Verification items for the finished model (mm, model axes). A direction names the side the tool comes from. Give positions to 0.01 mm unless a question says otherwise; leave off trailing zeros. Order: outer loops, then holes, each group sorted by start corner. A loop starts at its lowest first (then second) coordinate and runs counter-clockwise, first axis right, second up. Notation, with made-up numbers: M 61,79.5 L 98,79.5 A5 cw 98,87.5 Z; hole C -14,-33 d4. An arc over 180 degrees is marked long. Answer as a JSON object with one key per item and string values.
```python
from build123d import *

# Parameters (mm, degrees)
CROQUIS_TAPA_W                    = 110
CROQUIS_TAPA_H                    = 65
TAPA_DEPTH                        = 2.5
CROQUIS_PESTANA_W                 = 104.4
CROQUIS_PESTANA_H                 = 59.4
PESTANA_DEPTH                     = 4
CROQUIS_PESTANA_HUECO_W           = 101.4
CROQUIS_PESTANA_HUECO_H           = 56.4
PESTANA_HUECO_DEPTH               = 4
CROQUIS_POSTES_R                  = 2.5
POSTES_PCB_DEPTH                  = 29.9
VENTANA_LDR_Y_VENTILAS_DEPTH      = 71.535522965
VENTANA_LDR_Y_VENTILAS_DEPTH_BACK = 71.535522965
CROQUIS_VENTANA_Y_VENTILAS_R      = 3.5


with BuildPart() as part:
    # Croquis_tapa → Tapa (new body)
    with BuildSketch(Plane(origin=(0, 0, 0), x_dir=(1, 0, 0), z_dir=(0, 1, 0))):
        Rectangle(CROQUIS_TAPA_W, CROQUIS_TAPA_H)
    extrude(amount=TAPA_DEPTH)

    # Croquis_pestana → Pestana (add)
    with BuildSketch(Plane(origin=(0, 0, 0), x_dir=(1, 0, 0), z_dir=(0, 1, 0))):
        Rectangle(CROQUIS_PESTANA_W, CROQUIS_PESTANA_H)
    extrude(amount=-PESTANA_DEPTH)

    # Croquis_pestana_hueco → Pestana_hueco (cut)
    with BuildSketch(Plane(origin=(0, 0, 0), x_dir=(1, 0, 0), z_dir=(0, 1, 0))):
        Rectangle(CROQUIS_PESTANA_HUECO_W, CROQUIS_PESTANA_HUECO_H)
    extrude(amount=-PESTANA_HUECO_DEPTH, mode=Mode.SUBTRACT)

    # Croquis_postes → Postes_PCB (add)
    with BuildSketch(Plane(origin=(0, 0, 0), x_dir=(1, 0, 0), z_dir=(0, 1, 0))):
        with Locations(Location((-41, 22, 0), (0, 0, 270))):
            Circle(CROQUIS_POSTES_R)
        with Locations(Location((-41, -22, 0), (0, 0, 270))):
            Circle(CROQUIS_POSTES_R)
        with Locations(Location((41, 22, 0), (0, 0, 270))):
            Circle(CROQUIS_POSTES_R)
        with Locations(Location((41, -22, 0), (0, 0, 270))):
            Circle(CROQUIS_POSTES_R)
    extrude(amount=-POSTES_PCB_DEPTH)

    # Croquis_ventana_y_ventilas → Ventana_LDR_y_ventilas (cut, two sides: drawn at the far end of the back side and taken through both)
    with BuildSketch(Plane(origin=(0, 0, 0), x_dir=(1, 0, 0), z_dir=(0, 1, 0)).offset(-VENTANA_LDR_Y_VENTILAS_DEPTH_BACK)):
        with Locations(Location((33.46, -11, 0), (0, 0, 90))):
            Circle(CROQUIS_VENTANA_Y_VENTILAS_R)
        with BuildLine():
            Line((30, 0), (30, 8.68))
            ThreePointArc((30, 8.68), (31, 9.68), (32, 8.68))
            Line((32, 8.68), (32, 0))
            ThreePointArc((32, 0), (31, -1), (30, 0))
        make_face()
        with BuildLine():
            Line((34, 0), (34, 8.68))
            ThreePointArc((34, 8.68), (35, 9.68), (36, 8.68))
            Line((36, 8.68), (36, 0))
            ThreePointArc((36, 0), (35, -1), (34, 0))
        make_face()
        with BuildLine():
            Line((38, 0), (38, 8.68))
            ThreePointArc((38, 8.68), (39, 9.68), (40, 8.68))
            Line((40, 8.68), (40, 0))
            ThreePointArc((40, 0), (39, -1), (38, 0))
        make_face()
        with BuildLine():
            Line((-19, -15), (-19, 15))
            ThreePointArc((-19, 15), (-18, 16), (-17, 15))
            Line((-17, 15), (-17, -15))
            ThreePointArc((-17, -15), (-18, -16), (-19, -15))
        make_face()
        with BuildLine():
            Line((-23, -15), (-23, 15))
            ThreePointArc((-23, 15), (-22, 16), (-21, 15))
            Line((-21, 15), (-21, -15))
            ThreePointArc((-21, -15), (-22, -16), (-23, -15))
        make_face()
        with BuildLine():
            Line((-27, -15), (-27, 15))
            ThreePointArc((-27, 15), (-26, 16), (-25, 15))
            Line((-25, 15), (-25, -15))
            ThreePointArc((-25, -15), (-26, -16), (-27, -15))
        make_face()
        with BuildLine():
            Line((-31, -15), (-31, 15))
            ThreePointArc((-31, 15), (-30, 16), (-29, 15))
            Line((-29, 15), (-29, -15))
            ThreePointArc((-29, -15), (-30, -16), (-31, -15))
        make_face()
        with BuildLine():
            Line((-35, -15), (-35, 15))
            ThreePointArc((-35, 15), (-34, 16), (-33, 15))
            Line((-33, 15), (-33, -15))
            ThreePointArc((-33, -15), (-34, -16), (-35, -15))
        make_face()
        with BuildLine():
            Line((-39, -15), (-39, 15))
            ThreePointArc((-39, 15), (-38, 16), (-37, 15))
            Line((-37, 15), (-37, -15))
            ThreePointArc((-37, -15), (-38, -16), (-39, -15))
        make_face()
        with BuildLine():
            Line((-43, -15), (-43, 15))
            ThreePointArc((-43, 15), (-42, 16), (-41, 15))
            Line((-41, 15), (-41, -15))
            ThreePointArc((-41, -15), (-42, -16), (-43, -15))
        make_face()
    extrude(amount=VENTANA_LDR_Y_VENTILAS_DEPTH + VENTANA_LDR_Y_VENTILAS_DEPTH_BACK, mode=Mode.SUBTRACT)


solid = part.part
```
Q1. Section check C-C on y = -6.5. Record the cut outline in (x, z).
Resolved:
{"outline": "C -41,-22 d5; C -41,22 d5; C 41,-22 d5; C 41,22 d5"}
Q2. Material ranges on L1, parallel to X at y = -1, z = 25; L2, parallel to Y at x = -12, z = -27; L3, parallel to X at y = -8, z = 22.5, recorded low to high.
Resolved:
{"L1": "x = -52.2 to -50.7, 50.7 to 52.2", "L2": "y = 0 to 2.5", "L3": "x = -43.45 to -38.55, 38.55 to 43.45"}
Q3. Gauge pin test, flat ends, axial feed: pin 1 Ø12 at (x, z) = (39.5, -5.5) entering from +Y; pin 2 Ø3 at (x, z) = (-43.5, 9) entering from -Y; pin 3 Ø2 at (y, z) = (-1.5, -9) entering from +X. Record the tip position at first contact, or that the pin passes through.
Resolved:
{"pin 1": "stops at y = 2.5", "pin 2": "stops at y = 0", "pin 3": "stops at x = 52.2"}
Q4. Section check B-B on z = -6.5. Count the separate pieces of the cut face and the enclosed holes in it, then the cut area to 3 significant figures.
Resolved:
{"separate pieces": "11", "enclosed holes": "0", "area": "237 mm²"}
Q5. Tool access check on faces 4 (the face through (39.5, -14.7, -24)), 5 (the face through (-41, -29.9, 22)), 6 (the face through (-26, 1, 16)). Record the directions out of +Z, -Z, +X, -X, +Y, -Y that give a thin tool (end or side, any length) a straight path to the whole face; none if there is none.
Resolved:
{"face 4": "-Y", "face 5": "+Z, -Z, +X, -X, -Y", "face 6": "+Y, -Y"}
Q6. Section check A-A on x = 20. Record the cut outline in (y, z), then the cut area to 4 significant figures.
Resolved:
{"outline": "M -4,-29.7 L 0,-29.7 L 0,-32.5 L 2.5,-32.5 L 2.5,32.5 L 0,32.5 L 0,29.7 L -4,29.7 L -4,28.2 L 0,28.2 L 0,-28.2 L -4,-28.2 Z", "area": "174.5 mm²"}
Q7. Release check for a two-part mould opening along Z. For faces 1 (the face through (-41, -29.9, -22)), 2 (the face through (-1, 1, 32.5)), 3 (the face through (-43, 1, 0)) record: +Z half, -Z half, draft (parallel to the pull), parting line (faces both ways), or undercut.
Resolved:
{"face 1": "draft", "face 2": "+Z half", "face 3": "undercut"}
